from build123d import *

# Parameters (mm, degrees)
SKETCH1_W           = 20
SKETCH1_H           = 30
BOSS_EXTRUDE1_DEPTH = 3
SKETCH2_W           = 5
SKETCH2_H           = 30
BOSS_EXTRUDE2_DEPTH = 10
SKETCH3_R           = 1.5
CUT_EXTRUDE1_DEPTH  = 10
SKETCH4_R           = 1.6
CUT_EXTRUDE2_DEPTH  = 4


with BuildPart() as part:
    # Sketch1 → Boss-Extrude1 (new body)
    with BuildSketch(Plane(origin=(0, 0, 0), x_dir=(1, 0, 0), z_dir=(0, 1, 0))):
        Rectangle(SKETCH1_W, SKETCH1_H)
    extrude(amount=BOSS_EXTRUDE1_DEPTH)

    # Sketch2 → Boss-Extrude2 (add)
    with BuildSketch(Plane(origin=(0, 3, 0), x_dir=(1, 0, 0), z_dir=(0, 1, 0))):
        with Locations((-7.5, 0)):
            Rectangle(SKETCH2_W, SKETCH2_H)
    extrude(amount=BOSS_EXTRUDE2_DEPTH)

    # Sketch3 → Cut-Extrude1 (cut)
    with BuildSketch(Plane.ZY.offset(10)):
        with Locations((10, 7)):
            Circle(SKETCH3_R)
    extrude(amount=-CUT_EXTRUDE1_DEPTH, mode=Mode.SUBTRACT)

    # Sketch4 → Cut-Extrude2 (cut, through all)
    with BuildSketch(Plane(origin=(0, 3, 0), x_dir=(1, 0, 0), z_dir=(0, 1, 0))):
        with Locations((2.5, -7.5)):
            Circle(SKETCH4_R)
        with Locations((2.5, 7.5)):
            Circle(SKETCH4_R)
    extrude(amount=-CUT_EXTRUDE2_DEPTH, mode=Mode.SUBTRACT)


solid = part.part
Input: part model. Units: mm. Frame: model coordinates. A direction names the side the tool comes from. Coordinates: 2 decimals unless noted, no trailing zeros. Order: outer loops, then holes, each group sorted by start corner. A loop starts at its lowest first (then second) coordinate and runs counter-clockwise, first axis right, second up. Notation, with made-up numbers: M 52.5,29.25 L 65.5,29.25 A15 ccw 65.5,39.25 Z; hole C 7.5,37 d1. An arc over 180 degrees is marked long. Answer in a Markdown table with one row per item.
(1) Section query B-B, the plane z = -7.5. Output: boundary loops of the cut face in (x, y), plus the area to 3 significant figures.
Numbers:
| item | result |
|---|---|
| outline | M -10,0 L 0.9,0 L 0.9,3 L -5,3 L -5,13 L -10,13 Z; M 4.1,0 L 10,0 L 10,3 L 4.1,3 Z |
| area | 100 mm^2 |
(2) Access query for faces 4 (the flat face through (0, 0, 0)), 5 (the flat face through (-5, 8, 0)). Directions: +Z, -Z, +X, -X, +Y, -Y. A direction counts if a zero-diameter tool reaches every point of the face in a straight line with its end or side. Return the directions, or none.
Numbers:
| item | result |
|---|---|
| face 4 | +Z, -Z, +X, -X, -Y |
| face 5 | +Z, -Z, +X, +Y |
(3) Section query A-A, the plane x = 2.5. Output: boundary loops of the cut face in (y, z), plus the area to 3 significant figures.
Numbers:
| item | result |
|---|---|
| outline | M 0,-15 L 3,-15 L 3,-9.1 L 0,-9.1 Z; M 0,-5.9 L 3,-5.9 L 3,5.9 L 0,5.9 Z; M 0,9.1 L 3,9.1 L 3,15 L 0,15 Z |
| area | 70.8 mm^2 |
(4) Section query C-C, the plane y = 7. Output: boundary loops of the cut face in (x, z).
Numbers:
| item | result |
|---|---|
| outline | M -10,-15 L -5,-15 L -5,8.5 L -10,8.5 Z; M -10,11.5 L -5,11.5 L -5,15 L -10,15 Z |
(5) Section query D-D, the plane z = 6.25. Output: boundary loops of the cut face in (x, y).
Numbers:
| item | result |
|---|---|
| outline | M -10,0 L 1.5,0 L 1.5,3 L -5,3 L -5,13 L -10,13 Z; M 3.5,0 L 10,0 L 10,3 L 3.5,3 Z |
(6) Draft query along Z for faces 1 (the flat face through (10, 1, 0)), 2 (the flat face through (-5, 2, 15)), 3 (the cylindrical face through (-7.5, 6.1, 8.8)). Return one class per face: pulls with the +Z half, pulls with the -Z half, needs draft (parallel to the pull), parting line crosses it, or undercut.
Numbers:
| item | result |
|---|---|
| face 1 | needs draft |
| face 2 | pulls with the +Z half |
| face 3 | undercut |
(7) Contact query for a flat-ended pin moving along its axis: pin 1 Ø1.9 at (x, z) = (2.5, -7.5) entering from -Y. Output: stop coordinate, or through.
Numbers:
| item | result |
|---|---|
| pin 1 | passes through |
(8) Material intervals for line 1 (Z direction, x = 2.5, y = 2.05); line 2 (X direction, y = 1.3, z = -7.5); line 3 (Y direction, x = -8.9, z = 10), sorted ascending. Write a range as [from, to].
Numbers:
| item | result |
|---|---|
| line 1 | z = [-15, -9.1], [-5.9, 5.9], [9.1, 15] |
| line 2 | x = [-10, 0.9], [4.1, 10] |
| line 3 | y = [0, 5.5], [8.5, 13] |
